Part model, mm, in its own coordinate system. Face numbers are marked on the shaded views. A direction names the side the tool comes from. Give positions to 0.01 mm unless a question says otherwise; leave off trailing zeros. Loops run counter-clockwise (first coordinate to the right, second up) from the corner with the lowest first, then second, coordinate; pieces in that order, holes last. Notation, with made-up numbers: M 23,-4.75 L 51,-4.75 A31 cw 51,31.25 Z; hole C 47,49.5 d8. An arc over 180 degrees is marked long. Answer in a Markdown table with one row per item.
from build123d import *

# Parameters (mm, degrees)
DODANIE_WYCI_GNI_CIE1_DEPTH      = 4
DODANIE_WYCI_GNI_CIE1_DEPTH_BACK = 4
SZKIC1_W                         = 50
SZKIC1_H                         = 8
SZKIC1_R                         = 1.55
SZKIC2_R                         = 1.45
WYTNIJ_WYCI_GNI_CIE1_DEPTH       = 27.551836095
WYTNIJ_WYCI_GNI_CIE2_DEPTH       = 2.6
SZKIC4_R                         = 3
WYTNIJ_WYCI_GNI_CIE3_DEPTH       = 2.5
ZAOKR_GLENIE1_R                  = 4
SZKIC5_W                         = 6
SZKIC5_H                         = 4
WYTNIJ_WYCI_GNI_CIE4_DEPTH       = 2.5
SFAZOWANIE1_SIZE                 = 0.25


with BuildPart() as part:
    # Szkic1 → Dodanie-wyciągnięcie1 (new, two sides: drawn at the far end of the back side and taken through both)
    with BuildSketch(Plane.XY.offset(-DODANIE_WYCI_GNI_CIE1_DEPTH_BACK)):
        Rectangle(SZKIC1_W, SZKIC1_H)
        with Locations((-14, 0)):
            Circle(SZKIC1_R, mode=Mode.SUBTRACT)
        with Locations((14, 0)):
            Circle(SZKIC1_R, mode=Mode.SUBTRACT)
    extrude(amount=DODANIE_WYCI_GNI_CIE1_DEPTH + DODANIE_WYCI_GNI_CIE1_DEPTH_BACK)

    # Szkic2 → Wytnij-wyciągnięcie1 (cut, through all)
    with BuildSketch(Plane(origin=(0, 4, 0), x_dir=(1, 0, 0), z_dir=(0, 1, 0))):
        with Locations(Location((-21, 0, 0), (0, 0, 270))):
            Circle(SZKIC2_R)
        with Locations(Location((21, 0, 0), (0, 0, 270))):
            Circle(SZKIC2_R)
    extrude(amount=-WYTNIJ_WYCI_GNI_CIE1_DEPTH, mode=Mode.SUBTRACT)

    # Szkic3 → Wytnij-wyciągnięcie2 (cut)
    with BuildSketch(Plane(origin=(0, 4, 0), x_dir=(1, 0, 0), z_dir=(0, 1, 0))):
        Polygon((-17.766838493, 0), (-19.383419246, 2.8), (-22.616580754, 2.8), (-24.233161507, 0), (-22.616580754, -2.8), (-19.383419246, -2.8), align=None)
        Polygon((19.383419246, -2.8), (17.766838493, 0), (19.383419246, 2.8), (22.616580754, 2.8), (24.233161507, 0), (22.616580754, -2.8), align=None)
    extrude(amount=-WYTNIJ_WYCI_GNI_CIE2_DEPTH, mode=Mode.SUBTRACT)

    # Szkic4 → Wytnij-wyciągnięcie3 (cut)
    with BuildSketch(Plane.XY.offset(4)):
        with Locations((-14, 0)):
            Circle(SZKIC4_R)
        with Locations((14, 0)):
            Circle(SZKIC4_R)
    extrude(amount=-WYTNIJ_WYCI_GNI_CIE3_DEPTH, mode=Mode.SUBTRACT)

    # Zaokrąglenie1
    zaokr_glenie1_edges = [part.edges().sort_by_distance(p)[0] for p in [
        (25, 0, -4),
        (25, 0, 4),
        (-25, 0, 4),
        (-25, 0, -4),
    ]]
    fillet(zaokr_glenie1_edges, radius=ZAOKR_GLENIE1_R - 0.0001)  # a hair under: the kernel refuses the full size

    # Szkic5 → Wytnij-wyciągnięcie4 (cut)
    with BuildSketch(Plane.XY.offset(4)):
        with Locations((-14, 2)):
            Rectangle(SZKIC5_W, SZKIC5_H)
        with Locations((14, 2)):
            Rectangle(SZKIC5_W, SZKIC5_H)
    extrude(amount=-WYTNIJ_WYCI_GNI_CIE4_DEPTH, mode=Mode.SUBTRACT)

    # Sfazowanie1
    sfazowanie1_edges = [part.edges().sort_by_distance(p)[0] for p in [
        (19.00005, 4, 4),
        (0, 4, -4),
        (-23.828456414, 4, -2.828456414),
        (-23.828456414, 4, 2.828456414),
        (23.828456414, 4, 2.828456414),
        (23.828456414, 4, -2.828456414),
        (0, -4, -4),
        (0, -4, 4),
        (-23.828456414, -4, -2.828456414),
        (-23.828456414, -4, 2.828456414),
        (23.828456414, -4, 2.828456414),
        (23.828456414, -4, -2.828456414),
        (-14, -3, 4),
        (-15.55, 0, -4),
        (14, -3, 4),
        (0, 4, 4),
        (-19.00005, 4, 4),
        (-11, 2, 4),
        (-17, 2, 4),
        (17, 2, 4),
        (11, 2, 4),
        (12.45, 0, -4),
    ]]
    chamfer(sfazowanie1_edges, length=SFAZOWANIE1_SIZE)


solid = part.part
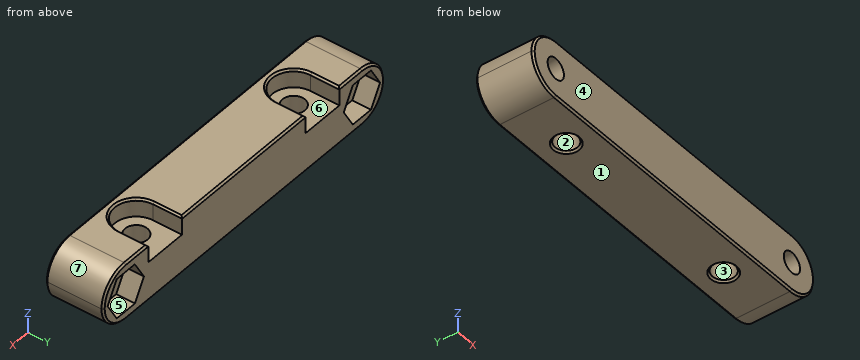
(1) Saw through at C-C (x = 18.5). Write the cut outline in (y, z).
Recorded:
| item | result |
|---|---|
| outline | M -4,-3.75 L -3.75,-4 L 3.75,-4 L 4,-3.75 L 4,-1.27 L 1.4,-1.27 L 1.4,1.27 L 4,1.27 L 4,3.75 L 3.75,4 L -3.75,4 L -4,3.75 Z |
(2) Pull direction Y, two halves, no side cores. Call the marked faces 1, 2, 3 and 4: +Y half, -Y half, draft (parallel to the pull), parting line (faces both ways), or undercut.
Recorded:
| item | result |
|---|---|
| face 1 | draft |
| face 2 | undercut |
| face 3 | undercut |
| face 4 | -Y half |
(3) Saw through at A-A (y = 3). Give the number of separate pieces and of enclosed holes in the cut face, plus the area to 3 significant figures.
Recorded:
| item | result |
|---|---|
| separate pieces | 1 |
| enclosed holes | 2 |
| area | 302 mm^2 |
(4) Drill centre lines: line 1 along X through (y, z) = (-1, -3); line 2 along X through (y, z) = (-0.9, 0); line 3 along Y through (x, z) = (-14, -0.95). Where is each one in solid material? Low to high.
Recorded:
| item | result |
|---|---|
| line 1 | x = -23.65 to -15.18, -12.82 to 12.82, 15.18 to 23.65 |
| line 2 | x = -25 to -22.45, -19.55 to -15.26, -12.74 to 12.74, 15.26 to 19.55, 22.45 to 25 |
| line 3 | y = -4 to -1.55, 1.55 to 4 |
(5) Which spindle directions (+Z, -Z, +X, -X, +Y, -Y) get a long thin tool onto all of the face, cutting with end or side? Do the marked faces 5, 6 and 7. Say none if no direction does.
Recorded:
| item | result |
|---|---|
| face 5 | +Y |
| face 6 | +Z, +Y |
| face 7 | +Z, +X, +Y, -Y |
(6) Pin check, flat tips, straight feed: pin 1 Ø1.8 at (y, z) = (1.5, 3) entering from +X; pin 2 Ø2 at (y, z) = (0.5, -2.5) entering from -X; pin 3 Ø1.1 at (y, z) = (1.5, 2.5) entering from -X; pin 4 Ø3 at (x, y) = (-14, 0) entering from -Z. Stop position of each tip, or through.
Recorded:
| item | result |
|---|---|
| pin 1 | stops at x = 24.4 |
| pin 2 | stops at x = -24.71 |
| pin 3 | stops at x = -24.49 |
| pin 4 | passes through |
